```python
from build123d import *

# Parameters (mm, degrees)
BOSS_EXTRUDE1_DEPTH = 30
SKETCH2_W           = 92
SKETCH2_H           = 5
CUT_EXTRUDE1_DEPTH  = 119.428248319
CHAMFER1_SIZE       = 4


with BuildPart() as part:
    # Sketch1 → Boss-Extrude1 (new body)
    with BuildSketch(Plane(origin=(0, 0, 0), x_dir=(1, 0, 0), z_dir=(0, 1, 0))):
        Polygon((-55, 55), (-42.5, 45.5), (-42.5, -45.5), (42.5, -45.5), (42.5, 45.5), (55, 55), (55, -55), (-55, -55), align=None)
    extrude(amount=BOSS_EXTRUDE1_DEPTH)

    # Sketch2 → Cut-Extrude1 (cut, through all)
    with BuildSketch(Plane(origin=(0, 0, 45.5), x_dir=(-1, 0, 0), z_dir=(0, 0, -1))):
        with Locations((0, 15)):
            Rectangle(SKETCH2_W, SKETCH2_H)
    extrude(amount=CUT_EXTRUDE1_DEPTH, mode=Mode.SUBTRACT)

    # Chamfer1
    # the kernel refuses this chamfer: 4 mm, written as the material it adds along each edge
    with BuildSketch(Plane(origin=(-46, 17.5, 55.786731952), x_dir=(-0.027495876610585623, -0.9996219169112968, 0), z_dir=(0, 0, -1))) as chamfer1_piece_1_section:
        Polygon((CHAMFER1_SIZE * 0.999621916911, -CHAMFER1_SIZE * 0.0274958766106), (-CHAMFER1_SIZE * 0.0274958766106, -CHAMFER1_SIZE * 0.999621916911), (0, 0), align=None)
    chamfer1_piece_1 = extrude(amount=114.233463904, mode=Mode.PRIVATE)
    chamfer1_piece_1 = split(chamfer1_piece_1, bisect_by=Plane(origin=(-22.386376136, 16.144806412, -30.213645864), z_dir=(-0.6050832675335592, 0, 0.7961621941231015)), keep=Keep.TOP, mode=Mode.PRIVATE)
    chamfer1_piece_1 = split(chamfer1_piece_1, bisect_by=Plane(origin=(-42.5, 16.144806412, -0.839947127), z_dir=(-1, 0, 0)), keep=Keep.TOP, mode=Mode.PRIVATE)
    chamfer1_piece_1 = split(chamfer1_piece_1, bisect_by=Plane(origin=(-44.710387176, 16.144806412, 55), z_dir=(0, 0, -1)), keep=Keep.TOP, mode=Mode.PRIVATE)
    add(chamfer1_piece_1)
    with BuildSketch(Plane(origin=(46, 17.5, 55.786731952), x_dir=(-0.9996219169112968, 0.02749587661058651, 0), z_dir=(0, 0, -1))) as chamfer1_piece_2_section:
        Polygon((CHAMFER1_SIZE * 0.999621916911, -CHAMFER1_SIZE * 0.0274958766106), (-CHAMFER1_SIZE * 0.0274958766106, -CHAMFER1_SIZE * 0.999621916911), (0, 0), align=None)
    chamfer1_piece_2 = extrude(amount=114.233463904, mode=Mode.PRIVATE)
    chamfer1_piece_2 = split(chamfer1_piece_2, bisect_by=Plane(origin=(22.386376136, 16.144806412, -30.213645864), z_dir=(0.6050832675335583, 0, 0.7961621941231022)), keep=Keep.TOP, mode=Mode.PRIVATE)
    chamfer1_piece_2 = split(chamfer1_piece_2, bisect_by=Plane(origin=(44.710387176, 16.144806412, 55), z_dir=(0, 0, -1)), keep=Keep.TOP, mode=Mode.PRIVATE)
    chamfer1_piece_2 = split(chamfer1_piece_2, bisect_by=Plane(origin=(42.5, 16.144806412, -0.839947127), z_dir=(1, 0, 0)), keep=Keep.TOP, mode=Mode.PRIVATE)
    add(chamfer1_piece_2)


solid = part.part
```
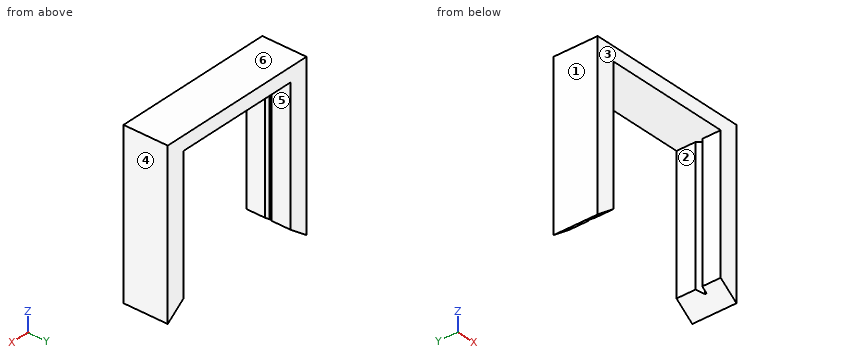
Geometry check sheet. Reference: the model listing, model coordinates, mm. Face numbers are marked on the shaded views. A direction names the side the tool comes from. Give positions to 0.01 mm unless a question says otherwise; leave off trailing zeros. Write each loop counter-clockwise with the first axis right and the second up, starting at its lowest first coordinate (ties: lowest second). Pieces come first, ordered by that corner, then holes. Notation, with made-up numbers: (6.25, -35) - (19.25, -35) arc R21 ccw to (19.25, -18) - close; hole circle Ø1 at (45.25, 20). An arc over 180 degrees is marked (long way). Use a Markdown table: item, result.
Q1. Section check B-B, the plane y = 5. Enter the section's corners in (x, z), then the cut area to 3 significant figures.
Computed:
| item | result |
|---|---|
| outline | (-55, -55) - (-42.5, -45.5) - (-42.5, 45.5) - (42.5, 45.5) - (42.5, -45.5) - (55, -55) - (55, 55) - (-55, 55) - close |
| area | 3,440 mm² |
Q2. Thickness scan on L1, parallel to X at y = 28, z = -40.5; L2, parallel to X at y = 12.75, z = -36.5; L3, parallel to Z at x = 15.5, y = 14.25. Record the ranges inside material, lowest first. Write a range as [from, to].
Computed:
| item | result |
|---|---|
| L1 | x = [-55, -42.5], [42.5, 55] |
| L2 | x = [-55, -46], [46, 55] |
| L3 | z = [45.5, 55] |
Q3. Section check C-C, the plane x = 44.5. Enter the section's corners in (y, z).
Computed:
| item | result |
|---|---|
| outline | (0, -47.02) - (12.5, -47.02) - (12.5, 45.5) - (15, 45.5) - (15, -47.02) - (30, -47.02) - (30, 55) - (0, 55) - close |
Q4. Set-up check for the marked faces 5 and 6: record each of +Z, -Z, +X, -X, +Y, -Y from which the full face is reachable in a straight line by a thin tool's end or side.
Computed:
| item | result |
|---|---|
| face 5 | -Z, +Y, -Y |
| face 6 | +Z, +X, -X, +Y, -Y |
Q5. Draft check along X on the marked faces 1, 2, 3 and 4. Enter one of: pulls with the +X half, pulls with the -X half, needs draft (parallel to the pull), parting line crosses it, or undercut.
Computed:
| item | result |
|---|---|
| face 1 | pulls with the -X half |
| face 2 | undercut |
| face 3 | needs draft |
| face 4 | pulls with the +X half |
Q6. Section check A-A, the plane z = 19. Enter the section's corners in (x, y), then the cut area to 3 significant figures.
Computed:
| item | result |
|---|---|
| outline | (-55, 0) - (-42.5, 0) - (-42.5, 12.5) - (-46, 12.5) - (-46, 13.5) - (-42.5, 17) - (-42.5, 30) - (-55, 30) - close; (42.5, 0) - (55, 0) - (55, 30) - (42.5, 30) - (42.5, 17) - (46, 13.5) - (46, 12.5) - (42.5, 12.5) - close |
| area | 731 mm² |
Q7. Section check D-D, the plane x = 20.5. Enter the section's corners in (y, z), then the cut area to 3 significant figures.
Computed:
| item | result |
|---|---|
| outline | (0, 45.5) - (30, 45.5) - (30, 55) - (0, 55) - close |
| area | 285 mm² |
Q8. Go/stop test with a flat-tipped pin: P1, Ø4, axis at x = 9, y = 12, coming from the -Z side. Record where the tip stops, or that it passes through.
Computed:
| item | result |
|---|---|
| P1 | stops at z = 45.5 |
